from build123d import *

# Parameters (mm, degrees)
BOSS_EXTRUDE1_DEPTH = 5.842
SKETCH3_R           = 2.38125
CUT_EXTRUDE2_DEPTH  = 30.127751029
FILLET1_R           = 3.175
SKETCH4_W           = 12.7
SKETCH4_H           = 0.1
BOSS_EXTRUDE2_DEPTH = 5.842


with BuildPart() as part:
    # Sketch1 → Boss-Extrude1 (new body)
    with BuildSketch(Plane(origin=(0, 0, 0), x_dir=(1, 0, 0), z_dir=(0, 1, 0))):
        Polygon((7.012, -12.7), (-7.012, -12.7), (-7.012, -6.45), (-12.854, -6.45), (-12.854, -12.7), (-25.554, -12.7), (-25.554, 12.7), (-12.854, 12.7), (-12.854, 6.45), (-7.012, 6.45), (-7.012, 12.7), (7.012, 12.7), (7.012, 6.45), (12.854, 6.45), (12.854, 12.7), (25.554, 12.7), (25.554, -12.7), (12.854, -12.7), (12.854, -6.45), (7.012, -6.45), align=None)
    extrude(amount=BOSS_EXTRUDE1_DEPTH)

    # Sketch3 → Cut-Extrude2 (cut, through all)
    with BuildSketch(Plane(origin=(0, 5.842, 0), x_dir=(1, 0, 0), z_dir=(0, 1, 0))):
        with Locations(Location((0, 0, 0), (0, 0, 270))):
            Circle(SKETCH3_R)
        with Locations(Location((-19.05, 0, 0), (0, 0, 270))):
            Circle(SKETCH3_R)
        with Locations(Location((19.05, 0, 0), (0, 0, 90))):
            Circle(SKETCH3_R)
    extrude(amount=-CUT_EXTRUDE2_DEPTH, mode=Mode.SUBTRACT)

    # Fillet1
    fillet1_edges = [part.edges().sort_by_distance(p)[0] for p in [
        (25.554, 2.921, -12.7),
        (-25.554, 2.921, -12.7),
    ]]
    fillet(fillet1_edges, radius=FILLET1_R)

    # Sketch4 → Boss-Extrude2 (add)
    with BuildSketch(Plane(origin=(0, 5.842, 0), x_dir=(1, 0, 0), z_dir=(0, 1, 0))):
        with Locations((-19.204, -12.75)):
            Rectangle(SKETCH4_W, SKETCH4_H)
        with Locations((19.204, -12.75)):
            Rectangle(SKETCH4_W, SKETCH4_H)
    extrude(amount=-BOSS_EXTRUDE2_DEPTH)


solid = part.part
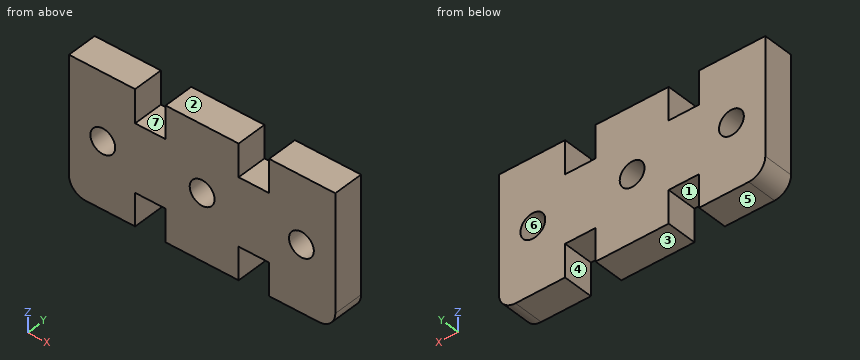
Input: part model. Units: mm. Frame: model coordinates. Face numbers are marked on the shaded views. A direction names the side the tool comes from. Coordinates: 2 decimals unless noted, no trailing zeros. Order: outer loops, then holes, each group sorted by start corner. A loop starts at its lowest first (then second) coordinate and runs counter-clockwise, first axis right, second up. Notation, with made-up numbers: M -31,62 L 21,62 A18 cw 21,66 Z; hole C -3,61 d2. An arc over 180 degrees is marked long. Answer in a Markdown table with one row per item.
(1) Section query C-C, the plane z = 8.75. Output: boundary loops of the cut face in (x, y).
Numbers:
| item | result |
|---|---|
| outline | M -25.55,0 L -12.85,0 L -12.85,5.84 L -25.55,5.84 Z; M -7.01,0 L 7.01,0 L 7.01,5.84 L -7.01,5.84 Z; M 12.85,0 L 25.55,0 L 25.55,5.84 L 12.85,5.84 Z |
(2) Draft query along Z for the marked faces 4, 5, 6 and 7. Return one class per face: pulls with the +Z half, pulls with the -Z half, needs draft (parallel to the pull), parting line crosses it, or undercut.
Numbers:
| item | result |
|---|---|
| face 4 | needs draft |
| face 5 | pulls with the -Z half |
| face 6 | undercut |
| face 7 | pulls with the +Z half |
(3) Section query A-A, the plane x = -19.05. Output: boundary loops of the cut face in (y, z).
Numbers:
| item | result |
|---|---|
| outline | M 0,-12.7 L 5.84,-12.7 L 5.84,-2.38 L 0,-2.38 Z; M 0,2.38 L 5.84,2.38 L 5.84,12.8 L 0,12.8 Z |
(4) Section query D-D, the plane x = 0. Output: boundary loops of the cut face in (y, z).
Numbers:
| item | result |
|---|---|
| outline | M 0,-12.7 L 5.84,-12.7 L 5.84,-2.38 L 0,-2.38 Z; M 0,2.38 L 5.84,2.38 L 5.84,12.7 L 0,12.7 Z |
(5) Contact query for flat-ended pins moving along their axis: pin 1 Ø2 at (x, y) = (-3, 5) entering from +Z; pin 2 Ø3 at (x, z) = (19.05, 0) entering from +Y; pin 3 Ø3 at (x, y) = (9, 4) entering from +Z; pin 4 Ø1.5 at (x, y) = (8.5, 1) entering from -Z. Output: stop coordinate, or through.
Numbers:
| item | result |
|---|---|
| pin 1 | stops at z = 12.7 |
| pin 2 | passes through |
| pin 3 | stops at z = 6.45 |
| pin 4 | stops at z = -6.45 |
(6) Access query for the marked faces 1, 2 and 3. Directions: +Z, -Z, +X, -X, +Y, -Y. A direction counts if a zero-diameter tool reaches every point of the face in a straight line with its end or side. Return the directions, or none.
Numbers:
| item | result |
|---|---|
| face 1 | -Z, +Y, -Y |
| face 2 | +Z, +Y, -Y |
| face 3 | -Z, +X, -X, +Y, -Y |
(7) Section query B-B, the plane y = 5.05. Give the number of separate pieces and of enclosed holes in the cut face, plus the area to 3 significant figures.
Numbers:
| item | result |
|---|---|
| separate pieces | 1 |
| enclosed holes | 3 |
| area | 1,100 mm^2 |
(8) Material intervals for line 1 (X direction, y = 2, z = 0); line 2 (X direction, y = 4, z = 11.25); line 3 (Z direction, x = 19.05, y = 4.4), sorted ascending. Write a range as [from, to].
Numbers:
| item | result |
|---|---|
| line 1 | x = [-25.55, -21.43], [-16.67, -2.38], [2.38, 16.67], [21.43, 25.55] |
| line 2 | x = [-25.55, -12.85], [-7.01, 7.01], [12.85, 25.55] |
| line 3 | z = [-12.7, -2.38], [2.38, 12.8] |
